Geometry check sheet. Reference: the model listing, model coordinates, mm. A direction names the side the tool comes from. Coordinates: 2 decimals unless noted, no trailing zeros. Loops run counter-clockwise (first coordinate to the right, second up) from the corner with the lowest first, then second, coordinate; pieces in that order, holes last.
from build123d import *

# Parameters (mm, degrees)
F0_R     = 11.1
F1_DEPTH = 6.5
F2_R     = 2.5
F3_SIZE  = 0.25


with BuildPart() as f1:
    # F0 (on Top) → F1 (new body)
    with BuildSketch(Plane.XY):
        with BuildLine():
            Line((14, 8.0829037687), (14, 0))
            ThreePointArc((14, 0), (12.124355653, -7), (7, -12.124355653))
            Line((7, -12.124355653), (0, -16.1658075373))
            Line((0, -16.1658075373), (20.2798002192, -27.874355653))
            ThreePointArc((20.2798002192, -27.874355653), (15.1554445662, -8.75), (34.2798002192, -3.625644347))
            Line((34.2798002192, -3.625644347), (14, 8.0829037687))
        make_face()
        with BuildLine():
            ThreePointArc((7, 12.124355653), (12.124355653, 7), (14, 0))
            Line((14, 0), (14, 8.0829037687))
            Line((14, 8.0829037687), (7, 12.124355653))
        make_face()
        with BuildLine():
            ThreePointArc((-7, 12.124355653), (0, 14), (7, 12.124355653))
            Line((7, 12.124355653), (14, 8.0829037687))
            Line((14, 8.0829037687), (14, 31.5))
            ThreePointArc((14, 31.5), (0, 17.5), (-14, 31.5))
            Line((-14, 31.5), (-14, 8.0829037687))
            Line((-14, 8.0829037687), (-7, 12.124355653))
        make_face()
        with BuildLine():
            Line((0, -16.1658075373), (7, -12.124355653))
            ThreePointArc((7, -12.124355653), (0, -14), (-7, -12.124355653))
            Line((-7, -12.124355653), (0, -16.1658075373))
        make_face()
        with BuildLine():
            ThreePointArc((-14, 0), (-12.124355653, 7), (-7, 12.124355653))
            Line((-7, 12.124355653), (-14, 8.0829037687))
            Line((-14, 8.0829037687), (-14, 0))
        make_face()
        with BuildLine():
            Line((0, -16.1658075373), (-7, -12.124355653))
            ThreePointArc((-7, -12.124355653), (-12.124355653, -7), (-14, 0))
            Line((-14, 0), (-14, 8.0829037687))
            Line((-14, 8.0829037687), (-34.2798002192, -3.625644347))
            ThreePointArc((-34.2798002192, -3.625644347), (-20.2798002192, -3.625644347), (-13.2798002192, -15.75))
            ThreePointArc((-13.2798002192, -15.75), (-15.1554445662, -22.75), (-20.2798002192, -27.874355653))
            Line((-20.2798002192, -27.874355653), (0, -16.1658075373))
        make_face()
        with BuildLine():
            ThreePointArc((-14, 31.5), (0, 17.5), (14, 31.5))
            ThreePointArc((14, 31.5), (0, 45.5), (-14, 31.5))
        make_face()
        Polygon((10.9696551146, 31.5), (5.4848275573, 22), (-5.4848275573, 22), (-10.9696551146, 31.5), (-5.4848275573, 41), (5.4848275573, 41), align=None, mode=Mode.SUBTRACT)
        with BuildLine():
            ThreePointArc((41.2798002192, -15.75), (39.4041558722, -8.75), (34.2798002192, -3.625644347))
            ThreePointArc((34.2798002192, -3.625644347), (15.1554445662, -8.75), (20.2798002192, -27.874355653))
            ThreePointArc((20.2798002192, -27.874355653), (34.2798002192, -27.874355653), (41.2798002192, -15.75))
        make_face()
        Polygon((16.3101451046, -15.75), (21.7949726619, -6.25), (32.7646277765, -6.25), (38.2494553338, -15.75), (32.7646277765, -25.25), (21.7949726619, -25.25), align=None, mode=Mode.SUBTRACT)
        with BuildLine():
            ThreePointArc((-34.2798002192, -3.625644347), (-39.4041558722, -22.75), (-20.2798002192, -27.874355653))
            ThreePointArc((-20.2798002192, -27.874355653), (-15.1554445662, -22.75), (-13.2798002192, -15.75))
            ThreePointArc((-13.2798002192, -15.75), (-20.2798002192, -3.625644347), (-34.2798002192, -3.625644347))
        make_face()
        Polygon((-21.7949726619, -6.25), (-16.3101451046, -15.75), (-21.7949726619, -25.25), (-32.7646277765, -25.25), (-38.2494553338, -15.75), (-32.7646277765, -6.25), align=None, mode=Mode.SUBTRACT)
        with BuildLine():
            ThreePointArc((7, -12.124355653), (12.124355653, -7), (14, 0))
            ThreePointArc((14, 0), (12.124355653, 7), (7, 12.124355653))
            ThreePointArc((7, 12.124355653), (0, 14), (-7, 12.124355653))
            ThreePointArc((-7, 12.124355653), (-12.124355653, 7), (-14, 0))
            ThreePointArc((-14, 0), (-12.124355653, -7), (-7, -12.124355653))
            ThreePointArc((-7, -12.124355653), (0, -14), (7, -12.124355653))
        make_face()
        Circle(F0_R, mode=Mode.SUBTRACT)
    extrude(amount=F1_DEPTH)

    # F2
    f2_edges = [f1.edges().sort_by_distance(p)[0] for p in [
        (-20.2798, -27.874356, 3.25),
        (0, -16.165808, 3.25),
        (-10.1399, -22.020082, 0),
        (-10.1399, -22.020082, 6.5),
        (-34.2798, -3.625644, 3.25),
        (-39.404156, -22.75, 0),
        (-39.404156, -22.75, 6.5),
        (20.2798, -27.874356, 3.25),
        (10.1399, -22.020082, 0),
        (10.1399, -22.020082, 6.5),
        (34.2798, -3.625644, 3.25),
        (39.404156, -22.75, 0),
        (39.404156, -22.75, 6.5),
        (14, 8.082904, 3.25),
        (24.1399, 2.22863, 0),
        (24.1399, 2.22863, 6.5),
        (14, 31.5, 3.25),
        (14, 19.791452, 0),
        (14, 19.791452, 6.5),
        (-14, 31.5, 3.25),
        (-14, 8.082904, 3.25),
        (-14, 19.791452, 0),
        (-14, 19.791452, 6.5),
        (-24.1399, 2.22863, 0),
        (-24.1399, 2.22863, 6.5),
    ]]
    fillet(f2_edges, radius=F2_R)

    # F3
    f3_edges = [f1.edges().sort_by_distance(p)[0] for p in [
        (19.052559, -20.5, 6.5),
        (19.052559, -11, 6.5),
        (27.2798, -6.25, 6.5),
        (35.507042, -11, 6.5),
        (35.507042, -20.5, 6.5),
        (27.2798, -25.25, 6.5),
        (-35.507042, -20.5, 6.5),
        (-35.507042, -11, 6.5),
        (-27.2798, -6.25, 6.5),
        (-19.052559, -11, 6.5),
        (-19.052559, -20.5, 6.5),
        (-27.2798, -25.25, 6.5),
        (0, 22, 6.5),
        (8.227241, 26.75, 6.5),
        (8.227241, 36.25, 6.5),
        (0, 41, 6.5),
        (-8.227241, 36.25, 6.5),
        (-8.227241, 26.75, 6.5),
    ]]
    chamfer(f3_edges, length=F3_SIZE)


solid = f1.part
1) Section check A-A on x = 0. Record the cut outline in (y, z), and give its area (3 significant figures).
Data:
outline: (-16.55, 2.5) arc R2.5 ccw to (-14.05, 0) - (-11.1, 0) - (-11.1, 6.5) - (-14.05, 6.5) arc R2.5 ccw to (-16.55, 4) - close; (11.1, 0) - (22, 0) - (22, 6.25) - (21.75, 6.5) - (11.1, 6.5) - close; (41, 0) - (43, 0) arc R2.5 ccw to (45.5, 2.5) - (45.5, 4) arc R2.5 ccw to (43, 6.5) - (41.25, 6.5) - (41, 6.25) - close
area: 130 mm2
2) Access from +Z, -Z, +X, -X, +Y, -Y to the whole of each face (thin tool, end or side, straight path). Record for faces 1 (the flat face through (35.469, -10.934, 3.081)), 2 (the flat face through (8.37, 26.76, 6.37)), 3 (the cylindrical face through (-10.988, -21.687, 0.752)).
Data:
face 1: +Z, -Z
face 2: +Z
face 3: -Z, -Y
3) Depth check by flat-ended pin: pin 1 (2 mm diameter, centred on x = 29.5, z = 4, fed in from +Y); pin 2 (0.5 mm diameter, centred on y = 23, z = 3.5, fed in from +X); pin 3 (3 mm diameter, centred on x = 2, z = 3.5, fed in from -Y); pin 4 (3 mm diameter, centred on x = -1, y = -10, fed in from +Z). Enter the tip coordinate at first touch or a pass-through.
Data:
pin 1: stops at y = -0.29
pin 2: stops at x = 14
pin 3: stops at y = -18.19
pin 4: stops at z = 6.5
4) Material ranges on probe 1 along Y at (x, z) = (0, 4.25); probe 2 along Y at (x, z) = (0, 4); probe 3 along X at (y, z) = (-12, 6.25), recorded low to high.
Data:
probe 1: y = -16.54 to -11.1, 11.1 to 22, 41 to 45.49
probe 2: y = -16.55 to -11.1, 11.1 to 22, 41 to 45.5
probe 3: x = -39.3 to -36.08, -18.48 to 18.48, 36.08 to 39.3
5) Mould release check, pull along Y, two halves, no side actions. Record for faces 4 (the flat face through (18.99, -20.63, 6.37)), 5 (the flat face through (-10.9, -22.46, 3.24)), 6 (the flat face through (-8.29, 26.62, 6.37)), 7 (the cylindrical face through (-13.287, 20.359, 0.752)): +Y half, -Y half, draft (parallel to the pull), parting line (faces both ways), or undercut.
Data:
face 4: undercut
face 5: -Y half
face 6: undercut
face 7: draft
